Design review of the part built by this model. Coordinates are the model's own, in mm. A direction names the side the tool comes from. Coordinates: 2 decimals unless noted, no trailing zeros. Loops run counter-clockwise (first coordinate to the right, second up) from the corner with the lowest first, then second, coordinate; pieces in that order, holes last. Notation, with made-up numbers: M 63.5,13.5 L 74.5,13.5 A32 cw 74.5,46.5 Z; hole C 68.5,-8 d3. An arc over 180 degrees is marked long. One line per item, written item: value.
```python
from build123d import *

# Parameters (mm, degrees)
F0_W      = 50.8
F0_H      = 50.8
F0_R      = 20.3708
F1_DEPTH  = 5.842
F7_ANGLE  = 330
F9_DEPTH  = 2.7432
F11_DEPTH = 1.8796


with BuildPart() as f1:
    # F0 (on Front) → F1 (new body)
    with BuildSketch(Plane.XZ):
        Rectangle(F0_W, F0_H)
        Circle(F0_R, mode=Mode.SUBTRACT)
    extrude(amount=-F1_DEPTH)

    # F2 (on Right) → F3 (revolve)
    with BuildSketch(Plane.YZ):
        Polygon((7.0104, 4.7625), (31.242, 4.7625), (31.242, 7.9375), (5.842, 7.9375), (5.842, 20.3708), (1.5494, 20.3708), (1.5494, 5.55625), (7.0104, 5.55625), align=None)
    revolve(axis=Axis((0, 6.768076, 0), (0, 1, 0)))

    # F6 (on face) → F7 (revolve, cut)
    with BuildSketch(Plane(origin=(0, 0, 0), x_dir=(0, -1, 0), z_dir=(-0.965926, 0, -0.258819))):
        with BuildLine():
            Line((-1.5494, 20.3708), (-1.6637, 20.3708))
            ThreePointArc((-1.6637, 20.3708), (-2.085772, 20.195972), (-2.2606, 19.7739))
            Line((-2.2606, 19.7739), (-2.2606, 19.4564))
            ThreePointArc((-2.2606, 19.4564), (-2.085772, 19.034328), (-1.6637, 18.8595))
            Line((-1.6637, 18.8595), (-1.5494, 18.8595))
            Line((-1.5494, 18.8595), (-1.5494, 20.3708))
        make_face()
    revolve(axis=Axis((0, -7.841465, 0), (0, -1, 0)), revolution_arc=F7_ANGLE, mode=Mode.SUBTRACT)

    # F8 (on face) → F9 (cut)
    with BuildSketch(Plane.XZ):
        with BuildLine():
            Line((-3.4925, 19.812), (-3.4925, 21.59))
            ThreePointArc((-3.4925, 21.59), (-5.08, 23.1775), (-6.6675, 21.59))
            Line((-6.6675, 21.59), (-6.6675, 19.812))
            ThreePointArc((-6.6675, 19.812), (-5.08, 18.2245), (-3.4925, 19.812))
        make_face()
        with BuildLine():
            Line((3.4925, 21.59), (3.4925, 19.812))
            ThreePointArc((3.4925, 19.812), (5.08, 18.2245), (6.6675, 19.812))
            Line((6.6675, 19.812), (6.6675, 21.59))
            ThreePointArc((6.6675, 21.59), (5.08, 23.1775), (3.4925, 21.59))
        make_face()
    extrude(amount=-F9_DEPTH, mode=Mode.SUBTRACT)

    # F10 (on face) → F11 (join)
    with BuildSketch(Plane.XZ.offset(-1.5494)):
        with BuildLine():
            Line((3.4925, 19.940258), (3.4925, 20.069179))
            ThreePointArc((3.4925, 20.069179), (0, 20.3708), (-3.4925, 20.069179))
            Line((-3.4925, 20.069179), (-3.4925, 19.940258))
            ThreePointArc((-3.4925, 19.940258), (0, 20.2438), (3.4925, 19.940258))
        make_face()
    extrude(amount=F11_DEPTH)


solid = f1.part
```
(1) We need section A-A on x = 0. State the section outline as (y, z) points.
Reply:
outline: M -0.33,20.24 L 1.55,20.24 L 1.55,5.56 L 7.01,5.56 L 7.01,4.76 L 31.24,4.76 L 31.24,7.94 L 5.84,7.94 L 5.84,25.4 L 0,25.4 L 0,20.37 L -0.33,20.37 Z; M 0,-25.4 L 5.84,-25.4 L 5.84,-7.94 L 31.24,-7.94 L 31.24,-4.76 L 7.01,-4.76 L 7.01,-5.56 L 1.55,-5.56 L 1.55,-18.86 L 1.66,-18.86 A0.6 cw 2.26,-19.46 L 2.26,-19.77 A0.6 cw 1.66,-20.37 L 0,-20.37 Z
(2) To check wall thickness, follow line 1 along X through (y, z) = (13, 0); line 2 along X through (y, z) = (0.7, 0); line 3 along Y through (x, z) = (-13.5, 19). State the ranges of each line that lie inside material, in increasing order. Write a range as [from, to].
Reply:
line 1: x = [-7.94, -4.76], [4.76, 7.94]
line 2: x = [-25.4, -20.37], [20.37, 25.4]
line 3: y = [0, 5.84]
(3) Tool access review of faces 1 (the flat face through (-25.4, 3, 0)), 2 (the flat face through (6, 5.842, 6)), 3 (the flat face through (2, 7.01, 5)): name each direction out of +Z, -Z, +X, -X, +Y, -Y from which nothing blocks a thin tool from reaching the whole face with its end or side.
Reply:
face 1: +Z, -Z, -X, +Y, -Y
face 2: +Y
face 3: -Y
(4) Insertion check: pin 1 (14.5 mm diameter, centred on x = 0, z = 0, fed in from -Y); pin 2 (12 mm diameter, centred on x = 1.5, z = -15, fed in from +Y); pin 3 (2 mm diameter, centred on y = 9.5, z = -7.5, fed in from +X). Each pin has a flat end and moves straight along its axis. Give the tip position at first contact, or say it passes through.
Reply:
pin 1: stops at y = 1.55
pin 2: stops at y = 5.84
pin 3: stops at x = 4.56
(5) We need section B-B on y = 14. State the section outline as (x, z) points (1 decimal), then the cut area to 3 significant figures.
Reply:
outline: C 0,0 d15.9; hole C 0,0 d9.5
area: 127 mm2
